```python
from build123d import *

# Parameters (mm, degrees)
EXTRUDE_1_DEPTH = 2


with BuildPart() as part:
    # Model → 凸台-拉伸1 (new body)
    with BuildSketch(Plane.XY):
        with BuildLine():
            Line((-35.311080617, 12.168656155), (465.757096498, 9.433834614))
            Line((465.757096498, 9.433834614), (464.752347114, 17.616861673))
            Line((464.752347114, 17.616861673), (462.76725481, 17.373122986))
            Line((462.76725481, 17.373122986), (461.547077382, 27.310670661))
            ThreePointArc((461.547077382, 27.310670661), (459.358669596, 20.416173483), (452.765919761, 17.439788161))
            Line((452.765919761, 17.439788161), (393.370792837, 17.835693957))
            ThreePointArc((393.370792837, 17.835693957), (386.669478588, 21.553462885), (382.152114107, 27.744007013))
            Line((382.152114107, 27.744007013), (383.335527601, 18.105877549))
            Line((383.335527601, 18.105877549), (381.350435298, 17.862138863))
            Line((381.350435298, 17.862138863), (380.135743173, 27.755012331))
            ThreePointArc((380.135743173, 27.755012331), (377.947335387, 20.860515153), (371.354585551, 17.884129831))
            Line((371.354585551, 17.884129831), (302.634100804, 18.330933271))
            ThreePointArc((302.634100804, 18.330933271), (295.932786555, 22.048702198), (291.415422074, 28.239246326))
            Line((291.415422074, 28.239246326), (292.594356772, 18.637593727))
            Line((292.594356772, 18.637593727), (290.609264469, 18.39385504))
            Line((290.609264469, 18.39385504), (289.39905114, 28.250251644))
            ThreePointArc((289.39905114, 28.250251644), (287.210643354, 21.355754466), (280.617893518, 18.379369144))
            Line((280.617893518, 18.379369144), (201.427401733, 19.185275472))
            ThreePointArc((201.427401733, 19.185275472), (194.726087484, 22.903044399), (190.208723003, 29.093588528))
            Line((190.208723003, 29.093588528), (191.522738388, 19.198231962))
            Line((191.522738388, 19.198231962), (189.289509547, 18.924025939))
            Line((189.289509547, 18.924025939), (188.076491094, 28.803268444))
            ThreePointArc((188.076491094, 28.803268444), (185.888083308, 21.908771266), (179.295333472, 18.932385944))
            Line((179.295333472, 18.932385944), (91.685409222, 19.482287621))
            ThreePointArc((91.685409222, 19.482287621), (84.984094973, 23.200056549), (80.466730491, 29.390600677))
            Line((80.466730491, 29.390600677), (81.651505322, 19.741384012))
            Line((81.651505322, 19.741384012), (79.666413019, 19.497645325))
            Line((79.666413019, 19.497645325), (78.450359557, 29.401605995))
            ThreePointArc((78.450359557, 29.401605995), (76.261951771, 22.507108817), (69.669201936, 19.530723495))
            Line((69.669201936, 19.530723495), (6.328074304, 19.948166495))
            ThreePointArc((6.328074304, 19.948166495), (-0.373239945, 23.665935423), (-4.890604427, 29.856479551))
            Line((-4.890604427, 29.856479551), (-3.70346647, 20.188016775))
            Line((-3.70346647, 20.188016775), (-5.688558774, 19.944278089))
            Line((-5.688558774, 19.944278089), (-6.906975361, 29.867484869))
            ThreePointArc((-6.906975361, 29.867484869), (-9.095383147, 22.972987691), (-15.688132982, 19.996602369))
            Line((-15.688132982, 19.996602369), (-24.269679134, 20.11516851))
            ThreePointArc((-24.269679134, 20.11516851), (-30.970993383, 23.832937438), (-35.488357864, 30.023481566))
            Line((-35.488357864, 30.023481566), (-34.288766793, 20.253596312))
            Line((-34.288766793, 20.253596312), (-36.273859097, 20.009857625))
            Line((-36.273859097, 20.009857625), (-35.311080617, 12.168656155))
        make_face()
    extrude(amount=EXTRUDE_1_DEPTH)


solid = part.part
```
Work out the finished part from the listing and answer in its coordinate system (mm). A direction names the side the tool comes from. Round coordinates to 2 decimals unless told otherwise and drop trailing zeros. Write each loop counter-clockwise with the first axis right and the second up, starting at its lowest first coordinate (ties: lowest second). Pieces come first, ordered by that corner, then holes. Notation, with made-up numbers: (8.5, -21.75) -> (46.5, -21.75) arc R26 cw to (46.5, 16.25) -> close; hole circle Ø1 at (-8, 67). An arc over 180 degrees is marked (long way). Write each question's results on one line, items separated by ' | '.
1) The part is cut by section B-B (x = 404.5). Write down the section's boundary in (y, z).
Findings:
outline: (9.77, 0) -> (17.76, 0) -> (17.76, 2) -> (9.77, 2) -> close
2) The part is cut by section A-A (x = 253). Write down the section's boundary in (y, z), and give its area (3 significant figures).
Findings:
outline: (10.6, 0) -> (18.66, 0) -> (18.66, 2) -> (10.6, 2) -> close | area: 16.1 mm²
3) Flat-ended cylindrical pins translate along their axes: pin 1 (1 mm diameter, centred on x = 37.5, z = 1.5, fed in from +Y); pin 2 (2 mm diameter, centred on x = 264, y = 18, fed in from -Z). Find the tip coordinate at first contact, or state that the pin passes through.
Findings:
pin 1: stops at y = 19.75 | pin 2: stops at z = 0
4) Consider line 1 along Y through (x, z) = (129, 0.8); line 2 along Y through (x, z) = (200, 1); line 3 along X through (y, z) = (15.25, 0.3). Determine where each line is inside the solid, lowest interval first. Write a range as [from, to].
Findings:
line 1: y = [11.27, 19.25] | line 2: y = [10.88, 19.68] | line 3: x = [-35.69, 465.04]
5) Which of the six approach directions +Z, -Z, +X, -X, +Y, -Y give full straight-line access (tool end or side, diameter ignored) to faces 1 (the flat face through (211, 15, 2)), 2 (the cylindrical face through (296.01, 21.98, 0.99))?
Findings:
face 1: +Z, +X, -X, +Y, -Y | face 2: +Z, -Z, +Y
6) For a pull along X with two mould halves and no side action, classify faces 3 (the flat face through (211, 15, 0)), 4 (the cylindrical face through (386.751, 21.482, 0.986)) as +X half, -X half, draft (parallel to the pull), parting line (faces both ways), or undercut.
Findings:
face 3: draft | face 4: undercut
